```python
from build123d import *

# Parameters (mm, degrees)
SKETCH1_W               = 88
SKETCH1_H               = 20
BOSS_EXTRUDE1_DEPTH     = 40
SKETCH2_R               = 4.25
CUT_EXTRUDE1_DEPTH      = 21
SKETCH7_R               = 12.5
BOSS_EXTRUDE2_DEPTH     = 40
SKETCH4_R               = 8.2
CUT_EXTRUDE3_DEPTH      = 41
FILLET2_R               = 10
SKETCH9_W               = 27
SKETCH9_H               = 21
CUT_EXTRUDE4_DEPTH      = 89
SKETCH10_W              = 63.73864418
SKETCH10_H              = 16
CUT_EXTRUDE5_DEPTH      = 13.5
CUT_EXTRUDE5_DEPTH_BACK = 13.5
FILLET3_R               = 5
SKETCH11_W              = 20
SKETCH11_H              = 19
BOSS_EXTRUDE3_DEPTH     = 6
SKETCH12_R              = 1.6
CUT_EXTRUDE6_DEPTH      = 20
FILLET5_R               = 5
BOSS_EXTRUDE4_DEPTH     = 4


with BuildPart() as part:
    # Sketch1 → Boss-Extrude1 (new body)
    with BuildSketch(Plane(origin=(0, 0, 0), x_dir=(1, 0, 0), z_dir=(0, 1, 0))):
        Rectangle(SKETCH1_W, SKETCH1_H)
    extrude(amount=BOSS_EXTRUDE1_DEPTH)

    # Sketch2 → Cut-Extrude1 (cut, through all)
    with BuildSketch(Plane.XY.offset(10)):
        with Locations((-38, 20)):
            Circle(SKETCH2_R)
        with Locations((38, 20)):
            Circle(SKETCH2_R)
    extrude(amount=-CUT_EXTRUDE1_DEPTH, mode=Mode.SUBTRACT)

    # Sketch7 → Boss-Extrude2 (add)
    with BuildSketch(Plane(origin=(0, 40, 0), x_dir=(1, 0, 0), z_dir=(0, 1, 0))):
        Circle(SKETCH7_R)
    extrude(amount=-BOSS_EXTRUDE2_DEPTH)

    # Sketch4 → Cut-Extrude3 (cut, through all)
    with BuildSketch(Plane(origin=(0, 40, 0), x_dir=(1, 0, 0), z_dir=(0, 1, 0))):
        Circle(SKETCH4_R)
    extrude(amount=-CUT_EXTRUDE3_DEPTH, mode=Mode.SUBTRACT)

    # Fillet2
    fillet2_edges = [part.edges().sort_by_distance(p)[0] for p in [
        (7.5, 20, -10),
        (7.5, 20, 10),
        (-7.5, 20, -10),
        (-7.5, 20, 10),
    ]]
    fillet(fillet2_edges, radius=FILLET2_R)

    # Sketch9 → Cut-Extrude4 (cut, through all)
    with BuildSketch(Plane.ZY.offset(44)):
        with Locations((0, 29.5)):
            Rectangle(SKETCH9_W, SKETCH9_H)
    extrude(amount=-CUT_EXTRUDE4_DEPTH, mode=Mode.SUBTRACT)

    # Sketch10 → Cut-Extrude5 (cut, two sides)
    with BuildSketch(Plane.XY) as cut_extrude5_sk:
        with Locations((0, 13)):
            Rectangle(SKETCH10_W, SKETCH10_H)
    extrude(amount=CUT_EXTRUDE5_DEPTH, mode=Mode.SUBTRACT)
    extrude(cut_extrude5_sk.sketch, amount=-CUT_EXTRUDE5_DEPTH_BACK, mode=Mode.SUBTRACT)

    # Fillet3
    fillet3_edges = [part.edges().sort_by_distance(p)[0] for p in [
        (31.86932209, 5, 0),
        (-31.86932209, 5, 0),
    ]]
    fillet(fillet3_edges, radius=FILLET3_R)

    # Sketch11 → Boss-Extrude3 (add)
    with BuildSketch(Plane(origin=(44, 0, 0), x_dir=(0, 0, -1), z_dir=(1, 0, 0))):
        with Locations((0, 9.5)):
            Rectangle(SKETCH11_W, SKETCH11_H)
    boss_extrude3 = extrude(amount=BOSS_EXTRUDE3_DEPTH)

    # Sketch12 → Cut-Extrude6 (cut, through all)
    with BuildSketch(Plane(origin=(0, 19, 0), x_dir=(1, 0, 0), z_dir=(0, 1, 0))):
        with Locations((46.065338955, 5)):
            Circle(SKETCH12_R)
        with Locations((46.065338955, -5)):
            Circle(SKETCH12_R)
    cut_extrude6 = extrude(amount=-CUT_EXTRUDE6_DEPTH, mode=Mode.SUBTRACT)

    # Mirror1: Boss-Extrude3, Cut-Extrude6 across plane
    add(boss_extrude3.mirror(Plane(origin=(0, 0, 0), x_dir=(0, 0, 1), z_dir=(1, 0, 0))))
    add(cut_extrude6.mirror(Plane(origin=(0, 0, 0), x_dir=(0, 0, 1), z_dir=(1, 0, 0))), mode=Mode.SUBTRACT)

    # Fillet5
    fillet5_edges = [part.edges().sort_by_distance(p)[0] for p in [
        (50, 9.5, -10),
        (50, 9.5, 10),
        (-50, 9.5, 10),
        (-50, 9.5, -10),
    ]]
    fillet(fillet5_edges, radius=FILLET5_R)

    # Sketch13 → Boss-Extrude4 (add)
    with BuildSketch(Plane.XY.offset(10)):
        with BuildLine():
            Line((-42.13067791, 19), (-33.86932209, 19))
            ThreePointArc((-33.86932209, 19), (-38, 15.75), (-42.13067791, 19))
        make_face()
        with BuildLine():
            Line((33.86932209, 19), (42.13067791, 19))
            ThreePointArc((42.13067791, 19), (38, 15.75), (33.86932209, 19))
        make_face()
    extrude(amount=-BOSS_EXTRUDE4_DEPTH)


solid = part.part
```
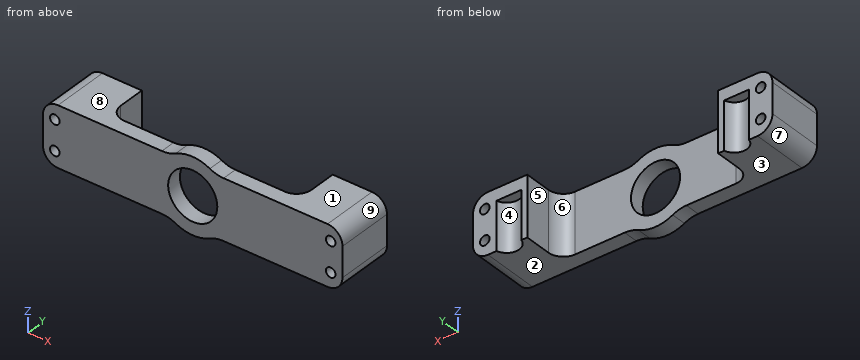
Can you work these out from the model? Positions are in its coordinate system, mm. Face numbers are marked on the shaded views. A direction names the side the tool comes from. Coordinates: 2 decimals unless noted, no trailing zeros. Loops run counter-clockwise (first coordinate to the right, second up) from the corner with the lowest first, then second, coordinate; pieces in that order, holes last. Notation, with made-up numbers: (-13, 20.5) -> (21, 20.5) arc R14 cw to (21, 42.5) -> close; hole circle Ø2 at (53.5, 40.5). An arc over 180 degrees is marked (long way). Answer as a JSON object with one key per item and string values.
1) If I drill on line 1 (X direction, y = 2.85, z = 0); line 2 (X direction, y = 2, z = -4.25); line 3 (X direction, y = 8.75, z = -5), over which ranges is the centre line in solid material (lowest first)?
Results:
{"line 1": "x = -50 to -8.2, 8.2 to 50", "line 2": "x = -50 to -47.48, -44.65 to -7.01, 7.01 to 44.65, 47.48 to 50", "line 3": "x = -50 to -47.67, -44.47 to -31.71, 31.71 to 44.47, 47.67 to 50"}
2) For P1, Ø2.5, axis at x = 38.5, y = 18, coming from the -Z side; P2, Ø12.5, axis at x = -12, z = -1.5, coming from the +Y side; P3, Ø5.5, axis at x = 36.5, y = 5, coming from the +Z side, each with a flat end and sliding along its axis, tell me the tip position at first contact or that it passes through.
Results:
{"P1": "stops at z = 6", "P2": "stops at y = 5", "P3": "stops at z = 10"}
3) Imagine slicing it at A-A (y = 14.25). Please give me the cut outline in (x, z).
Results:
{"outline": "(-50, -5) arc R5 ccw to (-45, -10) -> (-31.87, -10) -> (-31.87, 10) -> (-45, 10) arc R5 ccw to (-50, 5) -> close; (31.87, -10) -> (45, -10) arc R5 ccw to (50, -5) -> (50, 5) arc R5 ccw to (45, 10) -> (31.87, 10) -> close; hole circle Ø3.2 at (-46.07, -5); hole circle Ø3.2 at (-46.07, 5); hole circle Ø3.2 at (46.07, -5); hole circle Ø3.2 at (46.07, 5)"}
4) Imagine slicing it at C-C (x = 0). Please give me the cut outline in (y, z), then the cut area to 3 significant figures.
Results:
{"outline": "(0, -12.5) -> (5, -12.5) -> (5, -8.2) -> (0, -8.2) -> close; (0, 8.2) -> (5, 8.2) -> (5, 12.5) -> (0, 12.5) -> close", "area": "43.0 mm^2"}
5) For the marked faces 1, 2, 3, 4 and 5, which set-ups out of +Z, -Z, +X, -X, +Y, -Y let a thin tool reach every point of the face, with its end or its side?
Results:
{"face 1": "+Z, +X, +Y, -Y", "face 2": "-Z, +X, +Y, -Y", "face 3": "-Z, -X, +Y, -Y", "face 4": "-Z, +Y", "face 5": "+Z, -Z, +Y"}
6) Thinking about a two-plate mould opening in X: for the marked faces 6, 7, 8 and 9, which applies, pulls with the +X half, pulls with the -X half, needs draft (parallel to the pull), parting line crosses it, or undercut?
Results:
{"face 6": "undercut", "face 7": "pulls with the -X half", "face 8": "needs draft", "face 9": "pulls with the +X half"}
7) Imagine slicing it at B-B (z = 0). Please give me the cut outline in (x, y), then the cut area to 3 significant figures.
Results:
{"outline": "(-50, 0) -> (-8.2, 0) -> (-8.2, 5) -> (-26.87, 5) arc R5 cw to (-31.87, 10) -> (-31.87, 19) -> (-33.87, 19) arc R4.25 cw to (-42.13, 19) -> (-50, 19) -> close; (8.2, 0) -> (50, 0) -> (50, 19) -> (42.13, 19) arc R4.25 cw to (33.87, 19) -> (31.87, 19) -> (31.87, 10) arc R5 cw to (26.87, 5) -> (8.2, 5) -> close", "area": "896 mm^2"}
8) Imagine slicing it at D-D (y = 7.25). Please give me the cut outline in (x, z).
Results:
{"outline": "(-50, -5) arc R5 ccw to (-45, -10) -> (-31.05, -10) -> (-31.05, 10) -> (-45, 10) arc R5 ccw to (-50, 5) -> close; (31.05, -10) -> (45, -10) arc R5 ccw to (50, -5) -> (50, 5) arc R5 ccw to (45, 10) -> (31.05, 10) -> close; hole circle Ø3.2 at (-46.07, -5); hole circle Ø3.2 at (-46.07, 5); hole circle Ø3.2 at (46.07, -5); hole circle Ø3.2 at (46.07, 5)"}
